```python
from build123d import *

# Parameters (mm, degrees)
F1_DEPTH = 25


with BuildPart() as f1:
    # F0 (on Front) → F1 (new body)
    with BuildSketch(Plane.XZ):
        Polygon((-3.6047625217, 1.0570984669), (0, -2.4078239221), (3.464922389, 1.1969385996), (-11.515979737, 15.5966841781), (-15.9519963441, 12.9253440602), align=None)
        Polygon((-3.464922389, -6.0125864438), (0, -2.4078239221), (-3.6047625217, 1.0570984669), (-19.8503045149, -15.8440942143), (-15.3221144811, -18.3483206589), align=None)
        Polygon((3.464922389, 1.1969385996), (0, -2.4078239221), (3.6047625217, -5.8727463111), (19.8503045149, 11.0284463701), (15.3221144811, 13.5326728147), align=None)
        Polygon((3.6047625217, -5.8727463111), (0, -2.4078239221), (-3.464922389, -6.0125864438), (11.515979737, -20.4123320224), (15.9519963441, -17.7409919044), align=None)
        Polygon((-11.515979737, 15.5966841781), (3.464922389, 1.1969385996), (15.3221144811, 13.5326728147), (-0.4546866072, 22.2577223822), align=None)
        Polygon((-19.8503045149, -15.8440942143), (-3.6047625217, 1.0570984669), (-15.9519963441, 12.9253440602), (-21.5883330014, 9.5311790774), (-21.1336463941, -15.1343672269), align=None)
        Polygon((19.8503045149, 11.0284463701), (3.6047625217, -5.8727463111), (15.9519963441, -17.7409919044), (21.5883330014, -14.3468269216), (21.1336463941, 10.3187193827), align=None)
        Polygon((11.515979737, -20.4123320224), (-3.464922389, -6.0125864438), (-15.3221144811, -18.3483206589), (0.4546866072, -27.0733702264), align=None)
        with BuildLine():
            Line((22.8301708876, 21.3437454179), (15.3221144811, 13.5326728147))
            Line((15.3221144811, 13.5326728147), (19.8503045149, 11.0284463701))
            Line((19.8503045149, 11.0284463701), (27.1497799567, 18.6225199298))
            ThreePointArc((27.1497799567, 18.6225199298), (24.8510842543, 19.7626601145), (22.8301708876, 21.3437454179))
        make_face()
        with BuildLine():
            Line((-15.9519963441, 12.9253440602), (-11.515979737, 15.5966841781))
            Line((-11.515979737, 15.5966841781), (-22.7377914526, 26.3831663457))
            ThreePointArc((-22.7377914526, 26.3831663457), (-23.8506538485, 24.0646862159), (-25.4265858042, 22.0323842464))
            Line((-25.4265858042, 22.0323842464), (-15.9519963441, 12.9253440602))
        make_face()
        with BuildLine():
            Line((-15.3221144811, -18.3483206589), (-19.8503045149, -15.8440942143))
            Line((-19.8503045149, -15.8440942143), (-25.5164120913, -21.7388791308))
            ThreePointArc((-25.5164120913, -21.7388791308), (-23.2486379111, -22.9210064368), (-21.2450357109, -24.5102839214))
            Line((-21.2450357109, -24.5102839214), (-15.3221144811, -18.3483206589))
        make_face()
        with BuildLine():
            Line((22.3086725412, -23.8510725387), (15.9519963441, -17.7409919044))
            Line((15.9519963441, -17.7409919044), (11.515979737, -20.4123320224))
            Line((11.515979737, -20.4123320224), (19.572802502, -28.156605165))
            ThreePointArc((19.572802502, -28.156605165), (20.7252240198, -25.866894835), (22.3086725412, -23.8510725387))
        make_face()
        with BuildLine():
            ThreePointArc((44.2184696223, 30.4518900812), (26.6351729101, 42.0753321486), (22.8301708876, 21.3437454179))
            ThreePointArc((22.8301708876, 21.3437454179), (24.8510842543, 19.7626601145), (27.1497799567, 18.6225199298))
            ThreePointArc((27.1497799567, 18.6225199298), (38.7812636853, 20.0683193432), (44.2184696223, 30.4518900812))
        make_face()
        with BuildLine():
            Line((-29.2176456857, 32.6116465505), (-22.7377914526, 26.3831663457))
            ThreePointArc((-22.7377914526, 26.3831663457), (-22.2129285463, 28.3875102161), (-22.0362616439, 30.4518900812))
            ThreePointArc((-22.0362616439, 30.4518900812), (-45.4561166366, 34.9901269749), (-25.4265858042, 22.0323842464))
            Line((-25.4265858042, 22.0323842464), (-34.185892847, 30.4518900812))
            Line((-34.185892847, 30.4518900812), (-29.2176456857, 32.6116465505))
        make_face()
        with BuildLine():
            ThreePointArc((-25.4265858042, 22.0323842464), (-23.8506538485, 24.0646862159), (-22.7377914526, 26.3831663457))
            Line((-22.7377914526, 26.3831663457), (-29.2176456857, 32.6116465505))
            Line((-29.2176456857, 32.6116465505), (-34.185892847, 30.4518900812))
            Line((-34.185892847, 30.4518900812), (-25.4265858042, 22.0323842464))
        make_face()
        with BuildLine():
            Line((-34.1880838364, -30.7605291991), (-25.5164120913, -21.7388791308))
            ThreePointArc((-25.5164120913, -21.7388791308), (-41.7606868501, -41.7523739668), (-17.1078598825, -34.2254515881))
            ThreePointArc((-17.1078598825, -34.2254515881), (-18.1852212928, -28.9457568377), (-21.2450357109, -24.5102839214))
            Line((-21.2450357109, -24.5102839214), (-30.5833213146, -34.2254515881))
            Line((-30.5833213146, -34.2254515881), (-34.1880838364, -30.7605291991))
        make_face()
        with BuildLine():
            ThreePointArc((-21.2450357109, -24.5102839214), (-23.2486379111, -22.9210064368), (-25.5164120913, -21.7388791308))
            Line((-25.5164120913, -21.7388791308), (-34.1880838364, -30.7605291991))
            Line((-34.1880838364, -30.7605291991), (-30.5833213146, -34.2254515881))
            Line((-30.5833213146, -34.2254515881), (-21.2450357109, -24.5102839214))
        make_face()
        with BuildLine():
            ThreePointArc((44.4517230245, -32.7675244671), (36.3910799417, -20.832096116), (22.3086725412, -23.8510725387))
            Line((22.3086725412, -23.8510725387), (31.5849818289, -32.7675244671))
            Line((31.5849818289, -32.7675244671), (28.1200594399, -36.3722869888))
            Line((28.1200594399, -36.3722869888), (19.572802502, -28.156605165))
            ThreePointArc((19.572802502, -28.156605165), (29.2402615472, -45.4188214676), (44.4517230245, -32.7675244671))
        make_face()
        with BuildLine():
            Line((31.5849818289, -32.7675244671), (22.3086725412, -23.8510725387))
            ThreePointArc((22.3086725412, -23.8510725387), (20.7252240198, -25.866894835), (19.572802502, -28.156605165))
            Line((19.572802502, -28.156605165), (28.1200594399, -36.3722869888))
            Line((28.1200594399, -36.3722869888), (31.5849818289, -32.7675244671))
        make_face()
    extrude(amount=F1_DEPTH)


solid = f1.part
```
Geometry check sheet. Reference: the model listing, model coordinates, mm. A direction names the side the tool comes from. Coordinates: 2 decimals unless noted, no trailing zeros. Loops run counter-clockwise (first coordinate to the right, second up) from the corner with the lowest first, then second, coordinate; pieces in that order, holes last.
Item 1: Access from +Z, -Z, +X, -X, +Y, -Y to the whole of each face (thin tool, end or side, straight path). Record for faces 4 (the face through (-20.756, -12.325, 17.543)), 5 (the face through (-5.908, -12.325, 18.974)), 6 (the face through (5.91, -12.32, -23.79)), 7 (the face through (18.73, -12.32, -16.07)).
Item 2: Sectioned sample at A-A, the plane x = -28. Record the boundary of the cut face in (y, z), then the cut area to 3 significant figures.
Item 3: Sectioned sample at C-C, the plane z = 34. Record the boundary of the cut face in (x, y), then the cut area to 3 significant figures.
Item 4: Sectioned sample at D-D, the plane z = 7. Record the boundary of the cut face in (x, y).
Item 5: Thickness scan on line 1 (X direction, y = -6.5, z = 20.5); line 2 (Z direction, x = -19.5, y = -12.25); line 3 (X direction, y = -18.75, z = 24.5). Record the ranges inside material, lowest first.
Item 6: Sectioned sample at B-B, the plane y = -8.25. Record the boundary of the cut face in (x, z), then the cut area to 3 significant figures.
Item 7: Release check for a two-part mould opening along Z. For faces 1 (the face through (23.449, -12.325, 14.772)), 2 (the face through (7.544, -12.325, 17.834)), 3 (the face through (-7.54, -12.32, -22.65)) record: released by +Z, released by -Z, zero draft, split by the parting line, or undercut.
Item 8: Go/stop test with flat-tipped pins: pin 1 Ø6 at (y, z) = (-3, -21) entering from -X; pin 2 Ø5 at (y, z) = (-10.5, -13.5) entering from +X; pin 3 Ø12 at (y, z) = (-6, -22.5) entering from -X. Record where each tip stops, or that it passes through.
Check result:
1. face 4: +Y, -Y
1. face 5: +Z, +Y, -Y
1. face 6: -Z, +Y, -Y
1. face 7: +X, +Y, -Y
2. outline: (-25, -47.45) - (0, -47.45) - (0, -21) - (-25, -21) - close; (-25, 19.99) - (0, 19.99) - (0, 40.91) - (-25, 40.91) - close
2. area: 1,180 mm2
3. outline: (-45.81, -25) - (-22.57, -25) - (-22.57, 0) - (-45.81, 0) - close; (19.46, -25) - (43.71, -25) - (43.71, 0) - (19.46, 0) - close
3. area: 1,190 mm2
4. outline: (-21.54, -25) - (21.19, -25) - (21.19, 0) - (-21.54, 0) - close
5. line 1: x = -41.16 to -27.22, -23.83 to -16.62, -3.37 to 2.72, 22.02 to 39.37
5. line 2: z = -41.89 to -26.56, -22.69 to 10.79, 16.34 to 23.27
5. line 3: x = -44.78 to -20.78, 20.44 to 42.73
6. outline: (-25.52, -21.74) arc R13.48 ccw (long way) to (-21.25, -24.51) - (-15.32, -18.35) - (0.45, -27.07) - (11.52, -20.41) - (19.57, -28.16) arc R12.87 ccw (long way) to (22.31, -23.85) - (15.95, -17.74) - (21.59, -14.35) - (21.13, 10.32) - (19.85, 11.03) - (27.15, 18.62) arc R12.63 ccw (long way) to (22.83, 21.34) - (15.32, 13.53) - (-0.45, 22.26) - (-11.52, 15.6) - (-22.74, 26.38) arc R12.15 ccw (long way) to (-25.43, 22.03) - (-15.95, 12.93) - (-21.59, 9.53) - (-21.13, -15.13) - (-19.85, -15.84) - close
6. area: 3,850 mm2
7. face 1: undercut
7. face 2: released by +Z
7. face 3: released by -Z
8. pin 1: stops at x = -39.36
8. pin 2: stops at x = 21.59
8. pin 3: stops at x = -42.78
